```python
from build123d import *

# Parameters (mm, degrees)
SKETCH1_R           = 24.505905818
BOSS_EXTRUDE1_DEPTH = 0.2286
BOSS_EXTRUDE2_START = 63.5
BOSS_EXTRUDE2_DEPTH = 63.5
SKETCH4_W           = 63.5
SKETCH4_H           = 76.2
BOSS_EXTRUDE4_DEPTH = 14.929782549
SKETCH5_W           = 63.5
SKETCH5_H           = 50.8
BOSS_EXTRUDE5_DEPTH = 44.789347647
SKETCH7_W           = 63.5
SKETCH7_H           = 25.4
BOSS_EXTRUDE7_DEPTH = 22.41804
SKETCH8_W           = 63.5
SKETCH8_H           = 25.4
BOSS_EXTRUDE8_DEPTH = 22.41804
SKETCH9_W           = 48.26
SKETCH9_H           = 63.5
CUT_EXTRUDE1_DEPTH  = 179.030869421


with BuildPart() as part:
    # Sketch1 → Boss-Extrude1 (new body)
    with BuildSketch(Plane.YZ):
        with Locations(Location((0, 0, 0), (0, 0, 270))):
            Circle(SKETCH1_R)
    extrude(amount=BOSS_EXTRUDE1_DEPTH)

    # Sketch2 → Boss-Extrude2 (add)
    with BuildSketch(Plane(origin=(0, 0, 0), x_dir=(0, -1, 0), z_dir=(-1, 0, 0)).offset(BOSS_EXTRUDE2_START)):
        with BuildLine():
            Line((-24.505905818, 0), (-24.505905818, 76.2))
            Line((-24.505905818, 76.2), (24.505905818, 76.2))
            Line((24.505905818, 76.2), (24.505905818, 0))
            ThreePointArc((24.505905818, 0), (0, -24.505905818), (-24.505905818, 0))
        make_face()
    extrude(amount=-BOSS_EXTRUDE2_DEPTH)

    # Sketch4 → Boss-Extrude4 (add)
    with BuildSketch(Plane.XY.offset(76.2)):
        with Locations((-31.75, 0)):
            Rectangle(SKETCH4_W, SKETCH4_H)
    extrude(amount=BOSS_EXTRUDE4_DEPTH)

    # Sketch5 → Boss-Extrude5 (add)
    with BuildSketch(Plane(origin=(0, 38.1, 0), x_dir=(-1, 0, 0), z_dir=(0, 1, 0))):
        with Locations((31.75, 101.6)):
            Rectangle(SKETCH5_W, SKETCH5_H)
    boss_extrude5 = extrude(amount=BOSS_EXTRUDE5_DEPTH)

    # Mirror1: Boss-Extrude5 across plane
    add(boss_extrude5.mirror(Plane.ZX))

    # Sketch7 → Boss-Extrude7 (add)
    with BuildSketch(Plane.XZ.offset(-38.1)):
        with Locations((-31.75, 114.3)):
            Rectangle(SKETCH7_W, SKETCH7_H)
    extrude(amount=BOSS_EXTRUDE7_DEPTH)

    # Sketch8 → Boss-Extrude8 (add)
    with BuildSketch(Plane(origin=(0, -38.1, 0), x_dir=(-1, 0, 0), z_dir=(0, 1, 0))):
        with Locations((31.75, 114.3)):
            Rectangle(SKETCH8_W, SKETCH8_H)
    extrude(amount=BOSS_EXTRUDE8_DEPTH)

    # Sketch9 → Cut-Extrude1 (cut, through all)
    with BuildSketch(Plane.XZ.offset(24.505905818)):
        with Locations((-31.75, 44.45)):
            Rectangle(SKETCH9_W, SKETCH9_H)
    extrude(amount=-CUT_EXTRUDE1_DEPTH, mode=Mode.SUBTRACT)


solid = part.part
```
Could you check a few things on this model? Use its own coordinates, in mm. A direction names the side the tool comes from. Coordinates: 2 decimals unless noted, no trailing zeros. Write each loop counter-clockwise with the first axis right and the second up, starting at its lowest first coordinate (ties: lowest second). Pieces come first, ordered by that corner, then holes. Notation, with made-up numbers: (-36, -8) -> (-32, -8) arc R22 ccw to (-32, 24) -> close; hole circle Ø7 at (72.5, 66.5). An arc over 180 degrees is marked (long way). Write item = value, one per line. Start each with the question number.
(1) I want a section at A-A (y = 0). Please give me the cut outline in (x, z), plus the area to 3 significant figures.
(2) Which directions (+Z, -Z, +X, -X, +Y, -Y) give clear straight access to the entire face, cutting with the end or side of a thin tool? Please do faces 4 (the face through (-31, -50, 127)), 5 (the face through (-32, 15.682, 114)), 6 (the face through (-55.88, 0, 44)), 7 (the face through (-32, 1, 91.13)).
(3) I want a section at C-C (y = -19.5). Please give me the cut outline in (x, z).
(4) I want a section at B-B (z = 105). Please give me the cut outline in (x, y).
(5) I want a section at D-D (x = -26). Please give me the cut outline in (y, z), plus the area to 3 significant figures.
(6) Will these pins go through, and if not, where does the flat tip stop? pin 1 (18 mm diameter, centred on x = -32, y = 21.5, fed in from -Z); pin 2 (12 mm diameter, centred on x = -56, y = -15, fed in from -Z); pin 3 (19 mm diameter, centred on x = -36, y = -1.5, fed in from +Z); pin 4 (12 mm diameter, centred on x = -15, z = 43, fed in from +Y).
(7) We'd pull the mould along Y, two halves only. Please class faces 1 (the face through (-31, -38.1, 96)), 2 (the face through (-32, 24.506, 12)), 3 (the face through (-63.5, -1, 67)): released by +Y, released by -Y, zero draft, split by the parting line, or undercut.
(8) I need wall thicknesses on line 1 (X direction, y = -10, z = 68); line 2 (Z direction, x = -54, y = 31); line 3 (Z direction, x = -50.5, y = -1). Which ranges of each line are inside material? Lowest first, please. Write a range as [from, to].
Result set:
q1.outline = (-63.5, -24.51) -> (0.23, -24.51) -> (0.23, 24.51) -> (0, 24.51) -> (0, 91.13) -> (-63.5, 91.13) -> close; hole (-55.88, 12.7) -> (-7.62, 12.7) -> (-7.62, 76.2) -> (-55.88, 76.2) -> close
q1.area = 4,290 mm2
q2.face_4 = +Z, +X, -X, +Y, -Y
q2.face_5 = +Z, +X, -X
q2.face_6 = +Y, -Y
q2.face_7 = +X, -X
q3.outline = (-63.5, -14.84) -> (0.23, -14.84) -> (0.23, 14.84) -> (0, 14.84) -> (0, 91.13) -> (-63.5, 91.13) -> close; (-63.5, 101.6) -> (0, 101.6) -> (0, 127) -> (-63.5, 127) -> close; hole (-55.88, 12.7) -> (-7.62, 12.7) -> (-7.62, 76.2) -> (-55.88, 76.2) -> close
q4.outline = (-63.5, -82.89) -> (0, -82.89) -> (0, -15.68) -> (-63.5, -15.68) -> close; (-63.5, 15.68) -> (0, 15.68) -> (0, 82.89) -> (-63.5, 82.89) -> close
q5.outline = (-82.89, 76.2) -> (82.89, 76.2) -> (82.89, 127) -> (15.68, 127) -> (15.68, 101.6) -> (38.1, 101.6) -> (38.1, 91.13) -> (-38.1, 91.13) -> (-38.1, 101.6) -> (-15.68, 101.6) -> (-15.68, 127) -> (-82.89, 127) -> close; (-24.51, 0) arc R24.51 ccw to (24.51, 0) -> (24.51, 12.7) -> (-24.51, 12.7) -> close
q5.area = 8,390 mm2
q6.pin_1 = -21.08
q6.pin_2 = -22.79
q6.pin_3 = 91.13
q6.pin_4 = through
q7.face_1 = undercut
q7.face_2 = released by +Y
q7.face_3 = zero draft
q8.line_1 = [-63.5, -55.88], [-7.62, 0]
q8.line_2 = [76.2, 91.13], [101.6, 127]
q8.line_3 = [-24.49, 12.7], [76.2, 91.13]
